Work out the finished part from the listing and answer in its coordinate system (mm). Face numbers are marked on the shaded views. Give positions to 0.01 mm unless a question says otherwise; leave off trailing zeros. Loops run counter-clockwise (first coordinate to the right, second up) from the corner with the lowest first, then second, coordinate; pieces in that order, holes last. Notation, with made-up numbers: M -14,11.25 L 26,11.25 A11 cw 26,17.25 Z; hole C -35,51 d5. An arc over 180 degrees is marked long. Write item = value, one per line. Start each with the question number.
1. Section C-C on y = 5.25 is taken. Give the number of separate pieces and of enclosed holes in the cut face, plus the area to 3 significant figures.
2. Flat-ended cylindrical pins translate along their axes: pin 1 Ø6 at (y, z) = (2.5, 96.5) entering from +X; pin 2 Ø2 at (x, y) = (-30, 8) entering from -Z; pin 3 Ø4 at (y, z) = (9.5, 10) entering from +X; pin 4 Ø4.5 at (x, z) = (38.63, -118.88) entering from -Y. Find the tip coordinate at first contact, or state that the pin passes through.
3. Consider L1, parallel to Z at x = -100.5, y = 2; L2, parallel to X at y = 17.25, z = 1.5; L3, parallel to Z at x = -94.5, y = 13.75. Determine where each line is inside the solid, lowest interval first. Write a range as [from, to].
4. The mould has two halves that part along Z. Classify the marked faces 1, 2 and 3: released by +Z, released by -Z, zero draft, split by the parting line, or undercut.
5. Section B-B on z = -49 is taken. Determine the outline of the cut face in (x, y), plus the area to 3 significant figures.
6. Section A-A on x = 0 is taken. Determine the outline of the cut face in (y, z).
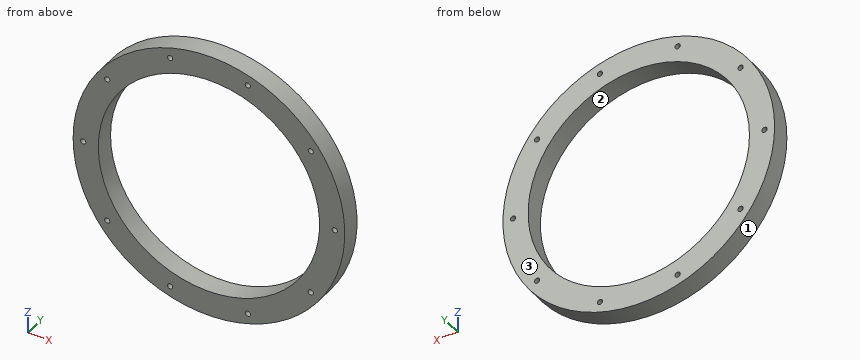
Autodesk Inventor part; units mm, degrees
ref_plane "YZ Plane" through (0, 0, 0) normal (1, 0, 0) x (0, 1, 0)
ref_plane "XZ Plane" through (0, 0, 0) normal (0, 1, 0) x (-1, 0, 0)
ref_plane "XY Plane" through (0, 0, 0) normal (0, 0, 1) x (1, 0, 0)
sketch "Sketch1" plane through (0, 0, 0) normal (0, 1, 0) x (-1, 0, 0)
  circle A0 centre (0, 0) radius 135
  circle A1 centre (0, 0) radius 110
  dimension "d0" = 270
  dimension "d1" = 220
extrude "Extrusion1" add sketch "Sketch1" along normal blind 20
sketch "Sketch2" plane through (0, 20, 0) normal (0, 1, 0) x (1, 0, 0)
  line L0 (-189, 0) -> (189, 0)
  point P0 (0, 0)
  point P1 (-125, 0)
  dimension "d11" = 125
hole "Hole1" at (-125, 20, 0) direction (0, -1, 0) diameter 5.2 end through all
pattern_circular "Circular Pattern1" count 10 over 360 about axis through (0, -10, 0) along (0, 1, 0) of "Hole1"
properties part number "Lower Ring (30mm)"
Verdict:
q1.separate_pieces = 1
q1.enclosed_holes = 11
q1.area = 19,000 mm2
q2.pin_1 = 97.38
q2.pin_2 = -131.85
q2.pin_3 = 134.76
q2.pin_4 = through
q3.L1 = [-90.14, -76], [-70.95, -44.72], [44.72, 70.95], [76, 90.14]
q3.L2 = [-134.99, -127.12], [-122.88, -109.99], [109.99, 122.88], [127.12, 134.99]
q3.L3 = [-96.41, -56.3], [56.3, 96.41]
q4.face_1 = split by the parting line
q4.face_2 = undercut
q4.face_3 = zero draft
q5.outline = M -125.79,0 L -98.48,0 L -98.48,20 L -125.79,20 Z; M 98.48,0 L 125.79,0 L 125.79,20 L 98.48,20 Z
q5.area = 1,090 mm2
q6.outline = M 0,-135 L 20,-135 L 20,-110 L 0,-110 Z; M 0,110 L 20,110 L 20,135 L 0,135 Z
